```python
from build123d import *

# Parameters (mm, degrees)
F3_DEPTH = 5
F4_R     = 2


with BuildPart() as f1:
    # F0 (on Front) → F1 (revolve)
    with BuildSketch(Plane.XZ):
        with BuildLine():
            Line((0, -25), (0, 0))
            Line((0, 0), (-9, 0))
            ThreePointArc((-9, 0), (-9.707107, -0.292893), (-10, -1))
            Line((-10, -1), (-10, -1.17097))
            Line((-10, -1.17097), (-4.791713, -6.379256))
            ThreePointArc((-4.791713, -6.379256), (-4.57494, -6.70368), (-4.49882, -7.086363))
            Line((-4.49882, -7.086363), (-4.49882, -25))
            Line((-4.49882, -25), (0, -25))
        make_face()
    revolve(axis=Axis((0, 0, -11.455107), (0, 0, -1)))

    # F2 (on face) → F3 (cut)
    with BuildSketch(Plane.XY):
        Polygon((-3.031089, -1.75), (0, -3.5), (3.031089, -1.75), (3.031089, 1.75), (0, 3.5), (-3.031089, 1.75), align=None)
    extrude(amount=-F3_DEPTH, mode=Mode.SUBTRACT)

    # F4
    f4_edges = [f1.edges().sort_by_distance(p)[0] for p in [
        (1.515544, -2.625, -5),
        (3.031089, 0, -5),
        (-1.515544, -2.625, -5),
        (-3.031089, 0, -5),
        (-1.515544, 2.625, -5),
        (1.515544, 2.625, -5),
    ]]
    fillet(f4_edges, radius=F4_R)


solid = f1.part
```
Here's how the part is built. I have some questions about the finished solid (model axes, mm). A direction names the side the tool comes from. Coordinates: 2 decimals unless noted, no trailing zeros. Loops run counter-clockwise (first coordinate to the right, second up) from the corner with the lowest first, then second, coordinate; pieces in that order, holes last. Notation, with made-up numbers: (-31.75, 18) - (15.25, 18) arc R6 cw to (15.25, 22) - close; hole circle Ø3 at (-17, -26). An arc over 180 degrees is marked (long way). Answer as CSV lines item,"result".
Q1. If we section it at A-A, the plane y = 0: Write out the boundary of the cut face in (x, z).
Response:
outline,"(-10, -1.17) - (-4.79, -6.38) arc R1 cw to (-4.5, -7.09) - (-4.5, -25) - (4.5, -25) - (4.5, -7.09) arc R1 cw to (4.79, -6.38) - (10, -1.17) - (10, -1) arc R1 ccw to (9, 0) - (3.03, 0) - (3.03, -3) arc R2 cw to (1.03, -5) - (-1.03, -5) arc R2 cw to (-3.03, -3) - (-3.03, 0) - (-9, 0) arc R1 ccw to (-10, -1) - close"
Q2. For pin 1 (4 mm diameter, centred on y = 7.5, z = -19.5, fed in from +X); pin 2 (0.9 mm diameter, centred on y = -0.5, z = -1.5, fed in from -X); pin 3 (0.6 mm diameter, centred on x = 0.5, y = 0.5, fed in from +Z); pin 4 (1.5 mm diameter, centred on y = -2, z = -19.5, fed in from -X), each with a flat end and sliding along its axis, tell me the tip position at first contact or that it passes through.
Response:
pin 1,"through"
pin 2,"x = -10"
pin 3,"z = -5"
pin 4,"x = -4.32"
Q3. We'd pull the mould along Y, two halves only. Please class faces 3 (the face through (0.98, -4.39, -16.17)), 4 (the face through (0, 0, -25)), 5 (the face through (-1.32, -2.335, -4.129)): pulls with the +Y half, pulls with the -Y half, needs draft (parallel to the pull), parting line crosses it, or undercut.
Response:
face 3,"parting line crosses it"
face 4,"needs draft"
face 5,"undercut"
Q4. For faces 1 (the face through (4, -3.07, -6.13)), 2 (the face through (-1.36, 2.31, -4.13)), which set-ups out of +Z, -Z, +X, -X, +Y, -Y let a thin tool reach every point of the face, with its end or its side?
Response:
face 1,"-Z"
face 2,"+Z"
Q5. If we section it at C-C, the plane z = -16.75: Write out the boundary of the cut face in (x, y).
Response:
outline,"circle Ø9 at (0, 0)"
Q6. If we section it at B-B, the plane z = -3.75: Write out the boundary of the cut face in (x, y).
Response:
outline,"circle Ø14.84 at (0, 0); hole (-2.89, -1.67) - (0, -3.33) - (2.89, -1.67) - (2.89, 1.67) - (0, 3.33) - (-2.89, 1.67) - close"
Q7. If I drill on L1, parallel to Z at x = -0.5, y = -1; L2, parallel to Y at x = 2.5, z = -2.5; L3, parallel to Y at x = 1.25, z = -18, over which ranges is the centre line in solid material (lowest first)? Write a range as [from, to].
Response:
L1,"[-25, -5]"
L2,"[-8.3, -2.06], [2.06, 8.3]"
L3,"[-4.32, 4.32]"
